Design review of the part built by this model. Coordinates are the model's own, in mm. Face numbers are marked on the shaded views. A direction names the side the tool comes from. Coordinates: 2 decimals unless noted, no trailing zeros. Order: outer loops, then holes, each group sorted by start corner. A loop starts at its lowest first (then second) coordinate and runs counter-clockwise, first axis right, second up.
from build123d import *

# Parameters (mm, degrees)
BOSS_EXTRU_1_DEPTH      = 5
BOSS_EXTRU_2_DEPTH      = 12
ESQUISSE4_W             = 3
ESQUISSE4_H             = 6
ENL_V_MAT_EXTRU_1_DEPTH = 41.844032186


with BuildPart() as part:
    # Esquisse1 → Boss.-Extru.1 (new body)
    with BuildSketch(Plane.XY):
        Polygon((2.690598923, 4.660254038), (-2.690598923, 4.660254038), (-5.381197846, 0), (-2.690598923, -4.660254038), (2.690598923, -4.660254038), (5.381197846, 0), align=None)
    boss_extru_1 = extrude(amount=BOSS_EXTRU_1_DEPTH)

    # Esquisse2 → Boss.-Extru.2 (add)
    with BuildSketch(Plane(origin=(0, 0, 0), x_dir=(-1, 0, 0), z_dir=(0, 0, -1))):
        Polygon((5.577350269, 9.660254038), (-5.577350269, 9.660254038), (-11.154700538, 0), (-5.577350269, -9.660254038), (5.577350269, -9.660254038), (11.154700538, 0), align=None)
    boss_extru_2 = extrude(amount=BOSS_EXTRU_2_DEPTH)

    # Esquisse4 → Enlèv. mat.-Extru.1 (cut, symmetric)
    with BuildSketch(Plane(origin=(-19.520725942, 14.490381057, 0), x_dir=(0, 0, 1), z_dir=(0.8660254037844387, 0.49999999999999983, 0))):
        with Locations((-10.5, 22.309401077)):
            Rectangle(ESQUISSE4_W, ESQUISSE4_H)
    enl_v_mat_extru_1 = extrude(amount=ENL_V_MAT_EXTRU_1_DEPTH, both=True, mode=Mode.SUBTRACT)

    # Symétrie1: Boss.-Extru.1, Boss.-Extru.2, Enlèv. mat.-Extru.1 across plane
    add(boss_extru_1.mirror(Plane(origin=(0, 0, -12), x_dir=(1, 0, 0), z_dir=(0, 0, -1))))
    add(boss_extru_2.mirror(Plane(origin=(0, 0, -12), x_dir=(1, 0, 0), z_dir=(0, 0, -1))))
    add(enl_v_mat_extru_1.mirror(Plane(origin=(0, 0, -12), x_dir=(1, 0, 0), z_dir=(0, 0, -1))), mode=Mode.SUBTRACT)


solid = part.part
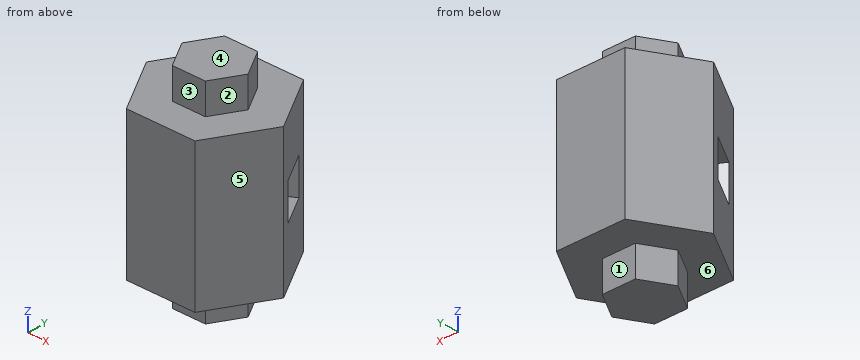
1. Add section A-A (z = -10.5). Give the boundary of the cut face in (x, y).
2. Add section B-B (x = 3.5). Give the boundary of the cut face in (y, z), and give its area (3 significant figures).
3. Insertion check: pin 1 (1 mm diameter, centred on x = -5.5, y = -6.5, fed in from -Z); pin 2 (8 mm diameter, centred on x = 6.5, y = 6.5, fed in from +Z); pin 3 (6 mm diameter, centred on y = 3.5, z = -2, fed in from -X). Each pin has a flat end and moves straight along its axis. Give the tip position at first contact, or say it passes through.
4. Mouldability with a two-part tool opening along Z and no side actions: class the marked faces 4, 5 and 6 as pulls with the +Z half, pulls with the -Z half, needs draft (parallel to the pull), parting line crosses it, or undercut.
5. To check wall thickness, follow line 1 (Z direction, x = -2.25, y = 0.25); line 2 (Z direction, x = -8.5, y = -1.75); line 3 (Z direction, x = 7.75, y = 0.75). State the ranges of each line that lie inside material, in increasing order.
6. Add section D-D (z = 1). Give the boundary of the cut face in (x, y), and give its area (3 significant figures).
7. Add section C-C (y = -1.5). Give the boundary of the cut face in (x, z).
8. For the marked faces 1, 2 and 3, list the 3-axis set-ups (+Z, -Z, +X, -X, +Y, -Y) from which the entire face can be reached by the end or side of a thin tool; tool diameter is ignored.
Solution:
1. outline: (-11.15, 0) - (-9.87, -2.23) - (6.87, 7.43) - (5.58, 9.66) - (-5.58, 9.66) - close; (-6.87, -7.43) - (-5.58, -9.66) - (5.58, -9.66) - (11.15, 0) - (9.87, 2.23) - close
2. outline: (-9.66, -24) - (-3.26, -24) - (-3.26, -29) - (3.26, -29) - (3.26, -24) - (9.66, -24) - (9.66, 0) - (3.26, 0) - (3.26, 5) - (-3.26, 5) - (-3.26, 0) - (-9.66, 0) - close; hole (-1.44, -15) - (5.48, -15) - (5.48, -9) - (-1.44, -9) - close
2. area: 487 mm2
3. pin 1: stops at z = -24
3. pin 2: stops at z = 0
3. pin 3: stops at x = -10.87
4. face 4: pulls with the +Z half
4. face 5: needs draft
4. face 6: pulls with the -Z half
5. line 1: z = -29 to -15, -9 to 5
5. line 2: z = -24 to -15, -9 to 0
5. line 3: z = -24 to 0
6. outline: (-5.38, 0) - (-2.69, -4.66) - (2.69, -4.66) - (5.38, 0) - (2.69, 4.66) - (-2.69, 4.66) - close
6. area: 75.2 mm2
7. outline: (-10.29, -24) - (-4.52, -24) - (-4.52, -29) - (4.52, -29) - (4.52, -24) - (10.29, -24) - (10.29, 0) - (4.52, 0) - (4.52, 5) - (-4.52, 5) - (-4.52, 0) - (-10.29, 0) - close; hole (-8.6, -15) - (3.4, -15) - (3.4, -9) - (-8.6, -9) - close
8. face 1: -Z, +X, -X, +Y
8. face 2: +Z, +X, -Y
8. face 3: +Z, +X, -X, -Y
